Build history of the part. All positions in model axes, mm. Coordinates: 2 decimals unless noted, no trailing zeros. Order: outer loops, then holes, each group sorted by start corner. A loop starts at its lowest first (then second) coordinate and runs counter-clockwise, first axis right, second up. Notation, with made-up numbers: M -4.5,47.25 L 29.5,47.25 A18 ccw 29.5,80.25 Z; hole C -37.5,46.25 d4. An arc over 180 degrees is marked long. Use a Markdown table: item, result. Add a question column.
from build123d import *

# Parameters (mm, degrees)
F1_DEPTH = 20
F3_DEPTH = 80
F4_R     = 2.5
F5_DEPTH = 5


with BuildPart() as f1:
    # F0 (on Top) → F1 (new body)
    with BuildSketch(Plane.XY):
        Polygon((-120, 90), (-200, 3.392654), (-196.32714, 0), (-117.81186, 85), (117.81186, 85), (196.32714, 0), (200, 3.392654), (120, 90), align=None)
    extrude(amount=F1_DEPTH)

    # F2 (on face) → F3 (join)
    with BuildSketch(Plane.XY.offset(20)):
        Polygon((-186.429383, 18.084093), (-200, 3.392654), (-196.32714, 0), (-182.756524, 14.691439), align=None)
        Polygon((200, 3.392654), (186.429383, 18.084093), (182.756524, 14.691439), (196.32714, 0), align=None)
    extrude(amount=F3_DEPTH)

    # F4 (on face) → F5 (join)
    with BuildSketch(Plane.XY.offset(100)):
        Polygon((196.32714, 0), (182.756524, 14.691439), (-182.756524, 14.691439), (-196.32714, 0), align=None)
        with Locations((-120, 7.345719)):
            Circle(F4_R, mode=Mode.SUBTRACT)
        with Locations((-40, 7.345719)):
            Circle(F4_R, mode=Mode.SUBTRACT)
        with Locations((40, 7.345719)):
            Circle(F4_R, mode=Mode.SUBTRACT)
        with Locations((120, 7.345719)):
            Circle(F4_R, mode=Mode.SUBTRACT)
    extrude(amount=-F5_DEPTH)


solid = f1.part
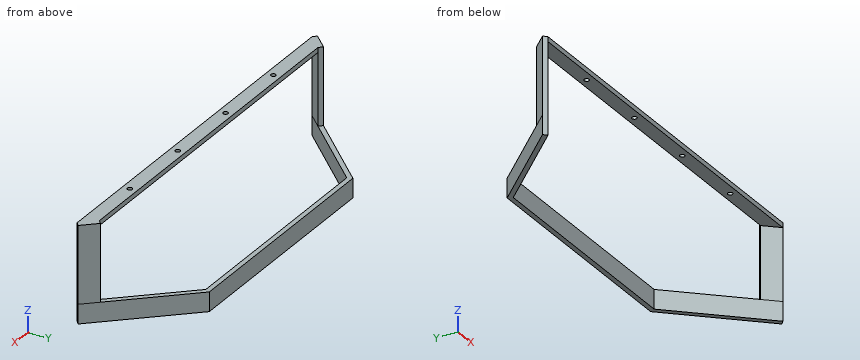
(1) Slice it at A-A on x = 7. Give the cut face in (y, z), and give its area (3 significant figures).
(2) Slice it at B-B on z = 68.5. Give the cut face in (x, y).
(3) Drill centre lines: line 1 along Y through (x, z) = (40, 96.25); line 2 along Z through (x, y) = (-112.5, 5); line 3 along X through (y, z) = (59, 6). Where is each one in solid material? Low to high. Write a range as from..to.
(4) Drop flat-ended pins along their axis: P1, Ø4.5, axis at x = -120, y = 7.35, coming from the +Z side; P2, Ø12, axis at x = 16, y = 8, coming from the -Z side; P3, Ø16, axis at x = -47, z = 7, coming from the -Y side; P4, Ø1.5, axis at x = 65.5, z = 98.5, coming from the +Y side. Give the stop position or say it passes through.
Solutions:
| question | item | result |
|---|---|---|
| 1 | outline | M 0,95 L 14.69,95 L 14.69,100 L 0,100 Z; M 85,0 L 90,0 L 90,20 L 85,20 Z |
| 1 | area | 173 mm² |
| 2 | outline | M -200,3.39 L -196.33,0 L -182.76,14.69 L -186.43,18.08 Z; M 182.76,14.69 L 196.33,0 L 200,3.39 L 186.43,18.08 Z |
| 3 | line 1 | 0..4.85, 9.85..14.69 |
| 3 | line 2 | 95..100 |
| 3 | line 3 | -148.63..-141.83, 141.83..148.63 |
| 4 | P1 | through |
| 4 | P2 | z = 95 |
| 4 | P3 | y = 85 |
| 4 | P4 | y = 14.69 |
